```python
from build123d import *

# Parameters (mm, degrees)
BOSS_EXTRUDE1_DEPTH = 25
CUT_EXTRUDE2_DEPTH  = 26
BOSS_EXTRUDE2_DEPTH = 0.4


with BuildPart() as part:
    # Sketch1 → Boss-Extrude1 (new body)
    with BuildSketch(Plane(origin=(0, 0, 0), x_dir=(1, 0, 0), z_dir=(0, 1, 0))):
        with BuildLine():
            ThreePointArc((1.451818925, -34.068556857), (1.641248992, -34.346908706), (1.964225605, -34.442038138))
            ThreePointArc((1.964225605, -34.442038138), (26.591847487, -21.978073076), (34.198225299, 4.555174015))
            ThreePointArc((34.198225299, 4.555174015), (23.590291339, 25.176355888), (2.324135821, 34.423627607))
            ThreePointArc((2.324135821, 34.423627607), (1.751838249, 34.289058819), (1.354061739, 33.856153382))
            ThreePointArc((1.354061739, 33.856153382), (0, 33.001534515), (-1.354061739, 33.856153382))
            ThreePointArc((-1.354061739, 33.856153382), (-1.751838249, 34.289058819), (-2.324135821, 34.423627607))
            ThreePointArc((-2.324135821, 34.423627607), (-23.590291339, 25.176355888), (-34.198225299, 4.555174015))
            ThreePointArc((-34.198225299, 4.555174015), (-26.591847487, -21.978073076), (-1.964225605, -34.442038138))
            ThreePointArc((-1.964225605, -34.442038138), (-1.641248992, -34.346908706), (-1.451818925, -34.068556857))
            ThreePointArc((-1.451818925, -34.068556857), (0, -32.945679925), (1.451818925, -34.068556857))
        make_face()
        with BuildLine():
            Line((-2.417, 3.787737139), (0, 3.787737139))
            Line((0, 3.787737139), (2.417, 3.787737139))
            ThreePointArc((2.417, 3.787737139), (0, -4.489512172), (-2.417, 3.787737139))
        make_face(mode=Mode.SUBTRACT)
    extrude(amount=BOSS_EXTRUDE1_DEPTH)

    # Sketch2 → Cut-Extrude2 (cut, through all)
    with BuildSketch(Plane(origin=(0, 0, 0), x_dir=(1, 0, 0), z_dir=(0, 1, 0))):
        with BuildLine():
            ThreePointArc((-21.79375, -3.005405287), (-15.556349186, -15.556349186), (-3.005405287, -21.79375))
            ThreePointArc((-3.005405287, -21.79375), (-1.991620962, -21.670338125), (-1.170937125, -21.0625))
            ThreePointArc((-1.170937125, -21.0625), (0, -20.5), (1.170937125, -21.0625))
            ThreePointArc((1.170937125, -21.0625), (1.991620962, -21.670338125), (3.005405287, -21.79375))
            ThreePointArc((3.005405287, -21.79375), (15.556349186, -15.556349186), (21.79375, -3.005405287))
            ThreePointArc((21.79375, -3.005405287), (21.670338125, -1.991620962), (21.0625, -1.170937125))
            ThreePointArc((21.0625, -1.170937125), (20.5, 0), (21.0625, 1.170937125))
            ThreePointArc((21.0625, 1.170937125), (21.670338125, 1.991620962), (21.79375, 3.005405287))
            ThreePointArc((21.79375, 3.005405287), (15.556349186, 15.556349186), (3.005405287, 21.79375))
            ThreePointArc((3.005405287, 21.79375), (1.991620962, 21.670338125), (1.170937125, 21.0625))
            ThreePointArc((1.170937125, 21.0625), (0, 20.5), (-1.170937125, 21.0625))
            ThreePointArc((-1.170937125, 21.0625), (-1.991620962, 21.670338125), (-3.005405287, 21.79375))
            ThreePointArc((-3.005405287, 21.79375), (-15.556349186, 15.556349186), (-21.79375, 3.005405287))
            ThreePointArc((-21.79375, 3.005405287), (-21.670338125, 1.991620962), (-21.0625, 1.170937125))
            ThreePointArc((-21.0625, 1.170937125), (-20.5, 0), (-21.0625, -1.170937125))
            ThreePointArc((-21.0625, -1.170937125), (-21.670338125, -1.991620962), (-21.79375, -3.005405287))
        make_face()
    extrude(amount=CUT_EXTRUDE2_DEPTH, mode=Mode.SUBTRACT)

    # Sketch2<2> → Boss-Extrude2 (add)
    with BuildSketch(Plane(origin=(0, 0, 0), x_dir=(1, 0, 0), z_dir=(0, 1, 0))):
        with BuildLine():
            ThreePointArc((-21.79375, -3.005405287), (-15.556349186, -15.556349186), (-3.005405287, -21.79375))
            ThreePointArc((-3.005405287, -21.79375), (-1.991620962, -21.670338125), (-1.170937125, -21.0625))
            ThreePointArc((-1.170937125, -21.0625), (0, -20.5), (1.170937125, -21.0625))
            ThreePointArc((1.170937125, -21.0625), (1.991620962, -21.670338125), (3.005405287, -21.79375))
            ThreePointArc((3.005405287, -21.79375), (15.556349186, -15.556349186), (21.79375, -3.005405287))
            ThreePointArc((21.79375, -3.005405287), (21.670338125, -1.991620962), (21.0625, -1.170937125))
            ThreePointArc((21.0625, -1.170937125), (20.5, 0), (21.0625, 1.170937125))
            ThreePointArc((21.0625, 1.170937125), (21.670338125, 1.991620962), (21.79375, 3.005405287))
            ThreePointArc((21.79375, 3.005405287), (15.556349186, 15.556349186), (3.005405287, 21.79375))
            ThreePointArc((3.005405287, 21.79375), (1.991620962, 21.670338125), (1.170937125, 21.0625))
            ThreePointArc((1.170937125, 21.0625), (0, 20.5), (-1.170937125, 21.0625))
            ThreePointArc((-1.170937125, 21.0625), (-1.991620962, 21.670338125), (-3.005405287, 21.79375))
            ThreePointArc((-3.005405287, 21.79375), (-15.556349186, 15.556349186), (-21.79375, 3.005405287))
            ThreePointArc((-21.79375, 3.005405287), (-21.670338125, 1.991620962), (-21.0625, 1.170937125))
            ThreePointArc((-21.0625, 1.170937125), (-20.5, 0), (-21.0625, -1.170937125))
            ThreePointArc((-21.0625, -1.170937125), (-21.670338125, -1.991620962), (-21.79375, -3.005405287))
        make_face()
    extrude(amount=BOSS_EXTRUDE2_DEPTH)


solid = part.part
```
The listing builds one solid part. Answer for the finished solid, in the listing's coordinates (mm). A direction names the side the tool comes from. Coordinates: 2 decimals unless noted, no trailing zeros. Write each loop counter-clockwise with the first axis right and the second up, starting at its lowest first coordinate (ties: lowest second). Pieces come first, ordered by that corner, then holes. Notation, with made-up numbers: M 87,36 L 122,36 A27 ccw 122,57 Z; hole C 14,59.25 d10. An arc over 180 degrees is marked long. Use a Markdown table: item, result. Add a question column.
1. Given P1, Ø2, axis at x = 10.5, y = 3.5, coming from the +Z side; P2, Ø8, axis at x = 17, y = 7.5, coming from the -Z side; P3, Ø12, axis at y = 12.5, z = -9.5, coming from the +X side, each flat-ended and moving along its own axis, determine where each tip first touches the part or whether it passes through.
2. Straight lines are drawn through the part: line 1 along Y through (x, z) = (20, -5.5); line 2 along X through (y, z) = (11.5, 17); line 3 along Z through (x, y) = (-6, 12.25). For each, find the intervals that lie inside material, in ascending order. Write a range as [from, to].
3. Section D-D (x = 28.5) is taken. Give the vertices of the cut face in (y, z).
4. Section C-C (z = 16) is taken. Give the vertices of the cut face in (x, y).
5. Section A-A (y = 12.75) is taken. Give the vertices of the cut face in (x, z).
6. Section B-B (x = 11) is taken. Give the vertices of the cut face in (y, z), plus the area to 3 significant figures.
7. For a pull along X with two mould halves and no side action, classify faces 3 (the flat face through (23, 25, 0)), 4 (the cylindrical face through (-21.676, 12.528, -2.005)) as +X half, -X half, draft (parallel to the pull), parting line (faces both ways), or undercut.
8. Which of the six approach directions +Z, -Z, +X, -X, +Y, -Y give full straight-line access (tool end or side, diameter ignored) to faces 1 (the cylindrical face through (15.7, 12.53, -15.41)), 2 (the flat face through (0, 0, 0))?
Data:
| question | item | result |
|---|---|---|
| 1 | P1 | stops at z = 33.16 |
| 1 | P2 | stops at z = -31.96 |
| 1 | P3 | stops at x = 34.32 |
| 2 | line 1 | y = [0, 0.4] |
| 2 | line 2 | x = [-30.02, -13.96], [13.96, 30.02] |
| 2 | line 3 | z = [-33.98, -21.17], [21.17, 33.97] |
| 3 | outline | M 0,-19.44 L 25,-19.44 L 25,19.44 L 0,19.44 Z |
| 4 | outline | M -30.56,0 L 30.56,0 L 30.56,25 L 15.1,25 L 15.1,0.4 L -15.1,0.4 L -15.1,25 L -30.56,25 Z |
| 5 | outline | M -2.32,-34.42 A1 ccw -1.35,-33.86 A1.5 cw 1.35,-33.86 A1 ccw 2.32,-34.42 A34.5 ccw 1.96,34.44 A0.5 ccw 1.45,34.07 A1.5 cw -1.45,34.07 A0.5 ccw -1.96,34.44 A34.5 ccw Z; hole M -21.79,-3.01 A22 ccw -3.01,-21.79 A2 ccw -1.17,-21.06 A1.5 cw 1.17,-21.06 A2 ccw 3.01,-21.79 A22 ccw 21.79,-3.01 A2 ccw 21.06,-1.17 A1.5 cw 21.06,1.17 A2 ccw 21.79,3.01 A22 ccw 3.01,21.79 A2 ccw 1.17,21.06 A1.5 cw -1.17,21.06 A2 ccw -3.01,21.79 A22 ccw -21.79,3.01 A2 ccw -21.06,1.17 A1.5 cw -21.06,-1.17 A2 ccw Z |
| 6 | outline | M 0,-32.7 L 25,-32.7 L 25,-19.05 L 0.4,-19.05 L 0.4,19.05 L 25,19.05 L 25,32.7 L 0,32.7 Z |
| 6 | area | 698 mm2 |
| 7 | face 3 | draft |
| 7 | face 4 | undercut |
| 8 | face 1 | +Y |
| 8 | face 2 | +Z, -Z, +X, -X, -Y |
